The model under review builds one solid part; all positions refer to its coordinate system, in mm. A direction names the side the tool comes from. Give positions to 0.01 mm unless a question says otherwise; leave off trailing zeros. Write each loop counter-clockwise with the first axis right and the second up, starting at its lowest first coordinate (ties: lowest second). Pieces come first, ordered by that corner, then holes. Notation, with made-up numbers: (83.25, -7.5) -> (139.25, -7.5) arc R31 cw to (139.25, 17.5) -> close; hole circle Ø7 at (1.25, 39.25). An arc over 180 degrees is marked (long way). Use CSV: the item, a comma, the result in double quotes.
```python
from build123d import *

# Parameters (mm, degrees)
SKETCH1_R           = 18.25
BOSS_EXTRUDE1_DEPTH = 90
SKETCH2_W           = 9
SKETCH2_H           = 6
CUT_EXTRUDE1_DEPTH  = 94.627586747
CHAMFER1_SIZE       = 2


with BuildPart() as part:
    # Sketch1 → Boss-Extrude1 (new body)
    with BuildSketch(Plane.XY):
        with Locations(Location((0, 0, 0), (0, 0, 180))):
            Circle(SKETCH1_R)
    extrude(amount=BOSS_EXTRUDE1_DEPTH)

    # Sketch2 → Cut-Extrude1 (cut, through all)
    with BuildSketch(Plane.XY.offset(90)):
        with Locations((0, 18.25)):
            Rectangle(SKETCH2_W, SKETCH2_H)
    extrude(amount=-CUT_EXTRUDE1_DEPTH, mode=Mode.SUBTRACT)

    # Chamfer1
    chamfer1_edges = [part.edges().sort_by_distance(p)[0] for p in [
        (0, -18.25, 90),
    ]]
    chamfer(chamfer1_edges, length=CHAMFER1_SIZE)


solid = part.part
```
Q1. Insertion check: pin 1 (4.5 mm diameter, centred on x = 0, z = 43.5, fed in from +Y); pin 2 (1.9 mm diameter, centred on y = 16, z = 49, fed in from -X); pin 3 (2 mm diameter, centred on x = 8.5, z = 29, fed in from -Y). Each pin has a flat end and moves straight along its axis. Give the tip position at first contact, or say it passes through.
Derived:
pin 1,"stops at y = 15.25"
pin 2,"stops at x = -10.32"
pin 3,"stops at y = -16.64"
Q2. Consider section B-B (z = 8). Write out the cut boundary in (x, y), then the cut area to 3 significant figures.
Derived:
outline,"(-4.5, 15.25) -> (-4.5, 17.69) arc R18.25 ccw (long way) to (4.5, 17.69) -> (4.5, 15.25) -> close"
area,"1,020 mm2"
Q3. The part is to be moulded in two halves that separate along X. For faces 1 (the flat face through (0, -1, 90)), 2 (the flat face through (4.5, 16, 46)), 3 (the cylindrical face through (-0.739, -18.235, 43.384)), say which applies: pulls with the +X half, pulls with the -X half, needs draft (parallel to the pull), parting line crosses it, or undercut.
Derived:
face 1,"needs draft"
face 2,"undercut"
face 3,"parting line crosses it"
Q4. Machinability: for faces 4 (the flat face through (-4.5, 16, 46)), 5 (the conical face through (0.671, -16.556, 89.681)), which of the approach directions +Z, -Z, +X, -X, +Y, -Y give a long, thin tool a straight path to every point of the face, cutting with its end or side? Answer none if there is none.
Derived:
face 4,"+Z, -Z, +Y"
face 5,"+Z"
Q5. To check wall thickness, follow probe 1 along Z at (x, y) = (-14, 10); probe 2 along Y at (x, z) = (0, 39.5); probe 3 along Y at (x, z) = (5.5, 8.5). State the ranges of each line that lie inside material, in increasing order.
Derived:
probe 1,"z = 0 to 89.05"
probe 2,"y = -18.25 to 15.25"
probe 3,"y = -17.4 to 17.4"
Q6. Consider section A-A (x = 0). Write out the cut boundary in (y, z).
Derived:
outline,"(-18.25, 0) -> (15.25, 0) -> (15.25, 90) -> (-16.25, 90) -> (-18.25, 88) -> close"
